from build123d import *

# Parameters (mm, degrees)
SKETCH1_W           = 122
SKETCH1_H           = 52
BOSS_EXTRUDE1_DEPTH = 6
SKETCH2_R           = 1.25
CUT_EXTRUDE1_DEPTH  = 53
SKETCH3_W           = 10
SKETCH3_H           = 10
CUT_EXTRUDE2_DEPTH  = 10


with BuildPart() as part:
    # Sketch1 → Boss-Extrude1 (new body)
    with BuildSketch(Plane.XY):
        with Locations((5.22260274, 1.88869863)):
            Rectangle(SKETCH1_W, SKETCH1_H)
    extrude(amount=-BOSS_EXTRUDE1_DEPTH)

    # Sketch2 → Cut-Extrude1 (cut, through all)
    with BuildSketch(Plane(origin=(0, 27.88869863, 0), x_dir=(1, 0, 0), z_dir=(0, 1, 0))):
        with Locations((-49.77739726, 3)):
            Circle(SKETCH2_R)
        with Locations((60.22260274, 3)):
            Circle(SKETCH2_R)
    extrude(amount=-CUT_EXTRUDE1_DEPTH, mode=Mode.SUBTRACT)

    # Sketch3 → Cut-Extrude2 (cut)
    with BuildSketch(Plane(origin=(0, 0, -6), x_dir=(-1, 0, 0), z_dir=(0, 0, -1))):
        with Locations((28.036600011, -19.11130137)):
            Rectangle(SKETCH3_W, SKETCH3_H)
    extrude(amount=-CUT_EXTRUDE2_DEPTH, mode=Mode.SUBTRACT)


solid = part.part
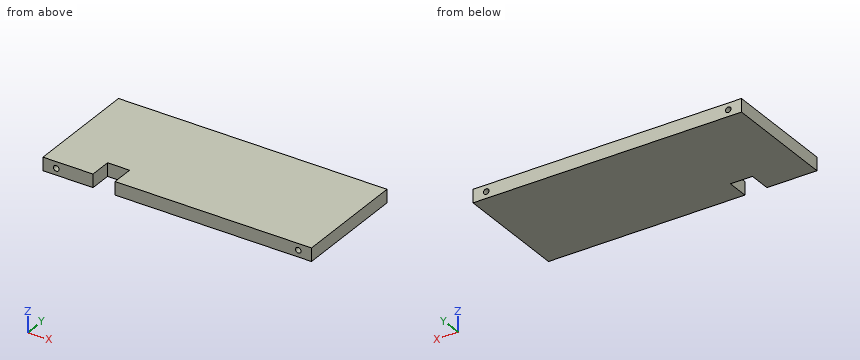
Verification items for the finished model (mm, model axes). Coordinates: 2 decimals unless noted, no trailing zeros. Order: outer loops, then holes, each group sorted by start corner. A loop starts at its lowest first (then second) coordinate and runs counter-clockwise, first axis right, second up.
Item 1: Depth check by flat-ended pin: pin 1 (3 mm diameter, centred on x = -26, z = -2, fed in from -Y). Enter the tip coordinate at first touch or a pass-through.
Filled in:
pin 1: stops at y = -14.11
Item 2: Section check A-A, the plane y = -17.5. Enter the section's corners in (x, z), then the cut area to 3 significant figures.
Filled in:
outline: (-55.78, -6) - (-33.04, -6) - (-33.04, 0) - (-55.78, 0) - close; (-23.04, -6) - (66.22, -6) - (66.22, 0) - (-23.04, 0) - close; hole circle Ø2.5 at (-49.78, -3); hole circle Ø2.5 at (60.22, -3)
area: 662 mm2
Item 3: Material ranges on L1, parallel to X at y = 17.5, z = -3; L2, parallel to X at y = 2, z = -3.95 (3 decimals); L3, parallel to X at y = -15.5, z = -3.35, recorded low to high.
Filled in:
L1: x = -55.78 to -51.03, -48.53 to 58.97, 61.47 to 66.22
L2: x = -55.777 to -50.59, -48.965 to 59.41, 61.035 to 66.223
L3: x = -55.78 to -50.98, -48.58 to -33.04, -23.04 to 59.02, 61.42 to 66.22
Item 4: Section check B-B, the plane z = -3. Enter the section's corners in (x, y), then the cut area to 3 significant figures.
Filled in:
outline: (-55.78, -24.11) - (-51.03, -24.11) - (-51.03, 27.89) - (-55.78, 27.89) - close; (-48.53, -24.11) - (-33.04, -24.11) - (-33.04, -14.11) - (-23.04, -14.11) - (-23.04, -24.11) - (58.97, -24.11) - (58.97, 27.89) - (-48.53, 27.89) - close; (61.47, -24.11) - (66.22, -24.11) - (66.22, 27.89) - (61.47, 27.89) - close
area: 5,980 mm2
